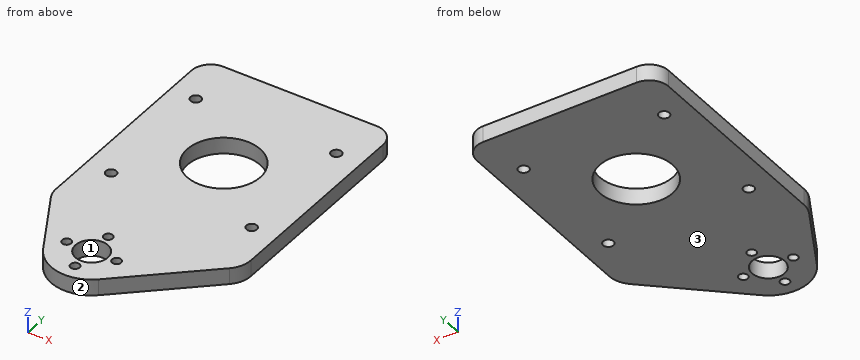
```python
from build123d import *

# Parameters (mm, degrees)
SKETCH1_W           = 304.8
SKETCH1_H           = 89.8
SKETCH1_R           = 14.2875
SKETCH1_R_2         = 2.54
SKETCH1_R_3         = 17.145
BOSS_EXTRUDE1_DEPTH = 6.35
SKETCH2_W           = 114.9
SKETCH2_H           = 89.8
SKETCH2_R           = 2.54
SKETCH2_R_2         = 17.145
CUT_EXTRUDE1_DEPTH  = 10
SKETCH4_R           = 6.35
SKETCH4_R_2         = 1.778
BOSS_EXTRUDE2_DEPTH = 6.35
FILLET1_R           = 10
FILLET2_R           = 7.5
SKETCH7_R           = 2.05
CUT_EXTRUDE2_DEPTH  = 10


with BuildPart() as part:
    # Sketch1 → Boss-Extrude1 (new body)
    with BuildSketch(Plane.XY):
        with Locations((152.4, 44.9)):
            Rectangle(SKETCH1_W, SKETCH1_H)
        with Locations((152.4, 44.9)):
            Circle(SKETCH1_R, mode=Mode.SUBTRACT)
        with Locations((109.401585406, 62.859439014)):
            Circle(SKETCH1_R_2, mode=Mode.SUBTRACT)
        with Locations((109.399439014, 26.938414594)):
            Circle(SKETCH1_R_2, mode=Mode.SUBTRACT)
        with Locations((73.478414594, 26.940560986)):
            Circle(SKETCH1_R_2, mode=Mode.SUBTRACT)
        with Locations((73.480560986, 62.861585406)):
            Circle(SKETCH1_R_2, mode=Mode.SUBTRACT)
        with Locations((91.44, 44.9)):
            Circle(SKETCH1_R_3, mode=Mode.SUBTRACT)
        with Locations((195.400560986, 62.861585406)):
            Circle(SKETCH1_R_2, mode=Mode.SUBTRACT)
        with Locations((231.321585406, 62.859439014)):
            Circle(SKETCH1_R_2, mode=Mode.SUBTRACT)
        with Locations((231.319439014, 26.938414594)):
            Circle(SKETCH1_R_2, mode=Mode.SUBTRACT)
        with Locations((195.398414594, 26.940560986)):
            Circle(SKETCH1_R_2, mode=Mode.SUBTRACT)
        with Locations((213.36, 44.9)):
            Circle(SKETCH1_R_3, mode=Mode.SUBTRACT)
    extrude(amount=BOSS_EXTRUDE1_DEPTH)

    # Sketch2 → Cut-Extrude1 (cut)
    with BuildSketch(Plane.XY.offset(6.35)):
        with Locations((247.35, 44.9)):
            Rectangle(SKETCH2_W, SKETCH2_H)
        with Locations((195.398414594, 26.940560986)):
            Circle(SKETCH2_R, mode=Mode.SUBTRACT)
        with Locations((231.319439014, 26.938414594)):
            Circle(SKETCH2_R, mode=Mode.SUBTRACT)
        with Locations((213.36, 44.9)):
            Circle(SKETCH2_R_2, mode=Mode.SUBTRACT)
        with Locations((195.400560986, 62.861585406)):
            Circle(SKETCH2_R, mode=Mode.SUBTRACT)
        with Locations((231.321585406, 62.859439014)):
            Circle(SKETCH2_R, mode=Mode.SUBTRACT)
        with Locations((57.45, 44.9)):
            Rectangle(SKETCH2_W, SKETCH2_H)
        with Locations((73.478414594, 26.940560986)):
            Circle(SKETCH2_R, mode=Mode.SUBTRACT)
        with Locations((109.399439014, 26.938414594)):
            Circle(SKETCH2_R, mode=Mode.SUBTRACT)
        with Locations((91.44, 44.9)):
            Circle(SKETCH2_R_2, mode=Mode.SUBTRACT)
        with Locations((73.480560986, 62.861585406)):
            Circle(SKETCH2_R, mode=Mode.SUBTRACT)
        with Locations((109.401585406, 62.859439014)):
            Circle(SKETCH2_R, mode=Mode.SUBTRACT)
    extrude(amount=-CUT_EXTRUDE1_DEPTH, mode=Mode.SUBTRACT)

    # Sketch4 → Boss-Extrude2 (add)
    with BuildSketch(Plane.XY.offset(6.35)):
        with BuildLine():
            Line((189.9, 0), (154.512001483, -31.80682216))
            ThreePointArc((154.512001483, -31.80682216), (141.221457874, -35.647397134), (129.96508312, -27.604848226))
            Line((129.96508312, -27.604848226), (114.9, 0))
            Line((114.9, 0), (189.9, 0))
        make_face()
        with Locations((143.9, -20)):
            Circle(SKETCH4_R, mode=Mode.SUBTRACT)
        with Locations((143.9, -29.779)):
            Circle(SKETCH4_R_2, mode=Mode.SUBTRACT)
        with Locations((134.121, -20)):
            Circle(SKETCH4_R_2, mode=Mode.SUBTRACT)
        with Locations((153.679, -20)):
            Circle(SKETCH4_R_2, mode=Mode.SUBTRACT)
        with Locations((143.9, -10.221)):
            Circle(SKETCH4_R_2, mode=Mode.SUBTRACT)
    extrude(amount=-BOSS_EXTRUDE2_DEPTH)

    # Fillet1
    fillet1_edges = [part.edges().sort_by_distance(p)[0] for p in [
        (189.9, 0, 3.175),
        (114.9, 0, 3.175),
    ]]
    fillet(fillet1_edges, radius=FILLET1_R)

    # Fillet2
    fillet2_edges = [part.edges().sort_by_distance(p)[0] for p in [
        (114.9, 89.8, 3.175),
        (189.9, 89.8, 3.175),
    ]]
    fillet(fillet2_edges, radius=FILLET2_R)

    # Sketch7 → Cut-Extrude2 (cut)
    with BuildSketch(Plane.XY.offset(6.35)):
        with Locations((179.9, 69.8)):
            Circle(SKETCH7_R)
        with Locations((124.9, 69.8)):
            Circle(SKETCH7_R)
        with Locations((124.9, 20)):
            Circle(SKETCH7_R)
        with Locations((179.9, 20)):
            Circle(SKETCH7_R)
    extrude(amount=-CUT_EXTRUDE2_DEPTH, mode=Mode.SUBTRACT)


solid = part.part
```
Build history of the part. All positions in model axes, mm. Face numbers are marked on the shaded views. Round coordinates to 2 decimals unless told otherwise and drop trailing zeros. Order: outer loops, then holes, each group sorted by start corner. A loop starts at its lowest first (then second) coordinate and runs counter-clockwise, first axis right, second up. Notation, with made-up numbers: (67, -3.75) -> (89, -3.75) arc R30 ccw to (89, 33.25) -> close; hole circle Ø6 at (-4.5, 80). An arc over 180 degrees is marked (long way). Answer in a Markdown table with one row per item.
1) Wall check: L1, parallel to Y at x = 143.9, z = 1.75 (3 decimals); L2, parallel to X at y = 44.5, z = 6; L3, parallel to Y at x = 179.9, z = 1.5. Give the ranges that are in metal, low to high.
Values:
| item | result |
|---|---|
| L1 | -35.875 to -31.557, -28.001 to -26.35, -13.65 to -11.999, -8.443 to 33.416, 56.384 to 89.8 |
| L2 | 114.9 to 138.12, 166.68 to 189.9 |
| L3 | -8.99 to 17.95, 22.05 to 67.75, 71.85 to 89.8 |
2) Band-saw the part on D-D on x = 159.5. Give the cut face in (y, z), and give its area (3 significant figures).
Values:
| item | result |
|---|---|
| outline | (-27.32, 0) -> (32.5, 0) -> (32.5, 6.35) -> (-27.32, 6.35) -> close; (57.3, 0) -> (89.8, 0) -> (89.8, 6.35) -> (57.3, 6.35) -> close |
| area | 586 mm2 |
3) Band-saw the part on A-A on y = 69.8. Give the cut face in (x, z).
Values:
| item | result |
|---|---|
| outline | (114.9, 0) -> (122.85, 0) -> (122.85, 6.35) -> (114.9, 6.35) -> close; (126.95, 0) -> (177.85, 0) -> (177.85, 6.35) -> (126.95, 6.35) -> close; (181.95, 0) -> (189.9, 0) -> (189.9, 6.35) -> (181.95, 6.35) -> close |
4) Band-saw the part on B-B on x = 124.9. Give the cut face in (y, z).
Values:
| item | result |
|---|---|
| outline | (-18.32, 0) -> (17.95, 0) -> (17.95, 6.35) -> (-18.32, 6.35) -> close; (22.05, 0) -> (67.75, 0) -> (67.75, 6.35) -> (22.05, 6.35) -> close; (71.85, 0) -> (89.8, 0) -> (89.8, 6.35) -> (71.85, 6.35) -> close |
5) Pin check, flat tips, straight feed: P1, Ø2.5, axis at x = 124.9, y = 69.8, coming from the +Z side; P2, Ø2, axis at y = -17, z = 2, coming from the -X side. Stop position of each tip, or through.
Values:
| item | result |
|---|---|
| P1 | through |
| P2 | x = 123.63 |
6) Band-saw the part on C-C on y = 44.9. Give the cut face in (x, z), and give its area (3 significant figures).
Values:
| item | result |
|---|---|
| outline | (114.9, 0) -> (138.11, 0) -> (138.11, 6.35) -> (114.9, 6.35) -> close; (166.69, 0) -> (189.9, 0) -> (189.9, 6.35) -> (166.69, 6.35) -> close |
| area | 295 mm2 |
7) Mould opens along Y. For the marked faces 1, 2 and 3 say: released by +Y, released by -Y, zero draft, split by the parting line, or undercut.
Values:
| item | result |
|---|---|
| face 1 | undercut |
| face 2 | released by -Y |
| face 3 | zero draft |
